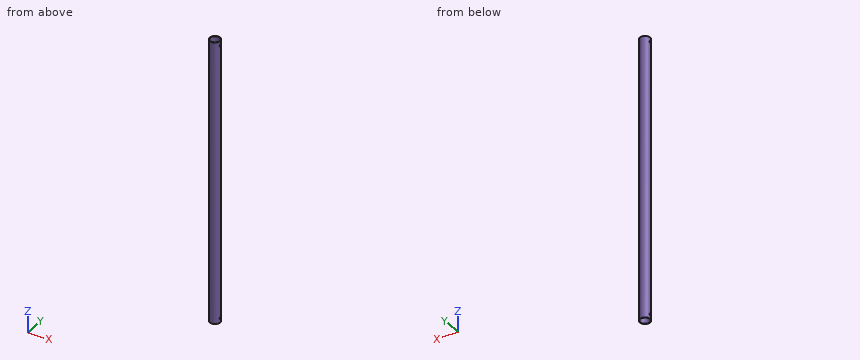
```python
from build123d import *

# Parameters (mm, degrees)
SKETCH2_R                                  = 17.5
SKETCH2_R_2                                = 15.9125
BOSS_EXTRUDE1_DEPTH                        = 474
SKETCH5_W                                  = 2.75
SKETCH5_H                                  = 17.5
MIRROR1_AT_THE_SECOND_PLANE_COPY_1_SKETC_W = 2.75
MIRROR1_AT_THE_SECOND_PLANE_COPY_1_SKETC_H = 17.5


with BuildPart() as part:
    # Sketch2 → Boss-Extrude1 (new body, symmetric)
    with BuildSketch(Plane.XY):
        Circle(SKETCH2_R)
        Circle(SKETCH2_R_2, mode=Mode.SUBTRACT)
    extrude(amount=BOSS_EXTRUDE1_DEPTH, both=True)

    # Sketch5 → M5 Clearance Hole1 (revolve, cut)
    with BuildSketch(Plane(origin=(0, 0, -459), x_dir=(0, 0, 1), z_dir=(0, 1, 0))):
        with Locations((1.375, 8.75)):
            Rectangle(SKETCH5_W, SKETCH5_H)
    m5_clearance_hole1 = revolve(axis=Axis((-6.35, 0, -459), (1, 0, 0)), mode=Mode.SUBTRACT)

    # Mirror1: M5 Clearance Hole1 across plane
    add(m5_clearance_hole1.mirror(Plane.XY), mode=Mode.SUBTRACT)

    # Mirror1 at the second plane: M5 Clearance Hole1 across plane
    add(m5_clearance_hole1.mirror(Plane(origin=(0, 0, 0), x_dir=(0, 0, 1), z_dir=(1, 0, 0))), mode=Mode.SUBTRACT)

    # Mirror1 at the second plane copy 1 sketc → Mirror1 at the second plane copy 1 (revolve, cut)
    with BuildSketch(Plane(origin=(0, 0, 459), x_dir=(0, 0, -1), z_dir=(0, 1, 0))):
        with Locations((1.375, 8.75)):
            Rectangle(MIRROR1_AT_THE_SECOND_PLANE_COPY_1_SKETC_W, MIRROR1_AT_THE_SECOND_PLANE_COPY_1_SKETC_H)
    revolve(axis=Axis((6.35, 0, 459), (-1, 0, 0)), mode=Mode.SUBTRACT)


solid = part.part
```
Can you work these out from the model? Positions are in its coordinate system, mm. Coordinates: 2 decimals unless noted, no trailing zeros. Write each loop counter-clockwise with the first axis right and the second up, starting at its lowest first coordinate (ties: lowest second). Pieces come first, ordered by that corner, then holes. Notation, with made-up numbers: M 10.5,60.5 L 67.5,60.5 A36 cw 67.5,94.5 Z; hole C -8.75,74.25 d6. An arc over 180 degrees is marked long. Write item = value, one per line. Start each with the question number.
Q1. If we section it at B-B, the plane z = -199.5: Write out the boundary of the cut face in (x, y) (1 decimal).
Q2. I'm going to push flat-ended pins straight in: pin 1 (1 mm diameter, centred on x = -3.5, z = 44, fed in from +Y); pin 2 (6.5 mm diameter, centred on y = 0, z = 459, fed in from +X); pin 3 (2 mm diameter, centred on y = 8.5, z = -306.5, fed in from -X); pin 4 (6 mm diameter, centred on x = 12.5, z = 303, fed in from +Y). Where does each tip first touch, or does it pass through?
Q3. If we section it at A-A, the plane x = 0: Write out the boundary of the cut face in (y, z).
Q4. If I drill on L1, parallel to Z at x = 16, y = 0; L2, parallel to X at y = 0, z = 119, over which ranges is the centre line in solid material (lowest first)? Write a range as [from, to].
Check sheet entries:
q1.outline = C 0,0 d35; hole C 0,0 d31.8
q2.pin_1 = 17.24
q2.pin_2 = 17.5
q2.pin_3 = -15.81
q2.pin_4 = 14.7
q3.outline = M -17.5,-474 L -15.91,-474 L -15.91,474 L -17.5,474 Z; M 15.91,-474 L 17.5,-474 L 17.5,474 L 15.91,474 Z
q4.L1 = [-474, -461.75], [-456.25, 456.25], [461.75, 474]
q4.L2 = [-17.5, -15.91], [15.91, 17.5]
